The figure shows three views and two pictorial views of one solid part (mm, origin at its lowest corner). Answer the questions. Round coordinates to 2 decimals unless told otherwise and drop trailing zeros. Write each loop counter-clockwise with the first axis right and the second up, starting at its lowest first coordinate (ties: lowest second). Pieces come first, ordered by that corner, then holes. Notation, with made-up numbers: M 74,14 L 98,14 A20 cw 98,33 Z; hole C 73,-10 d11. An arc over 180 degrees is marked long. Answer in a Markdown table with one row per item.
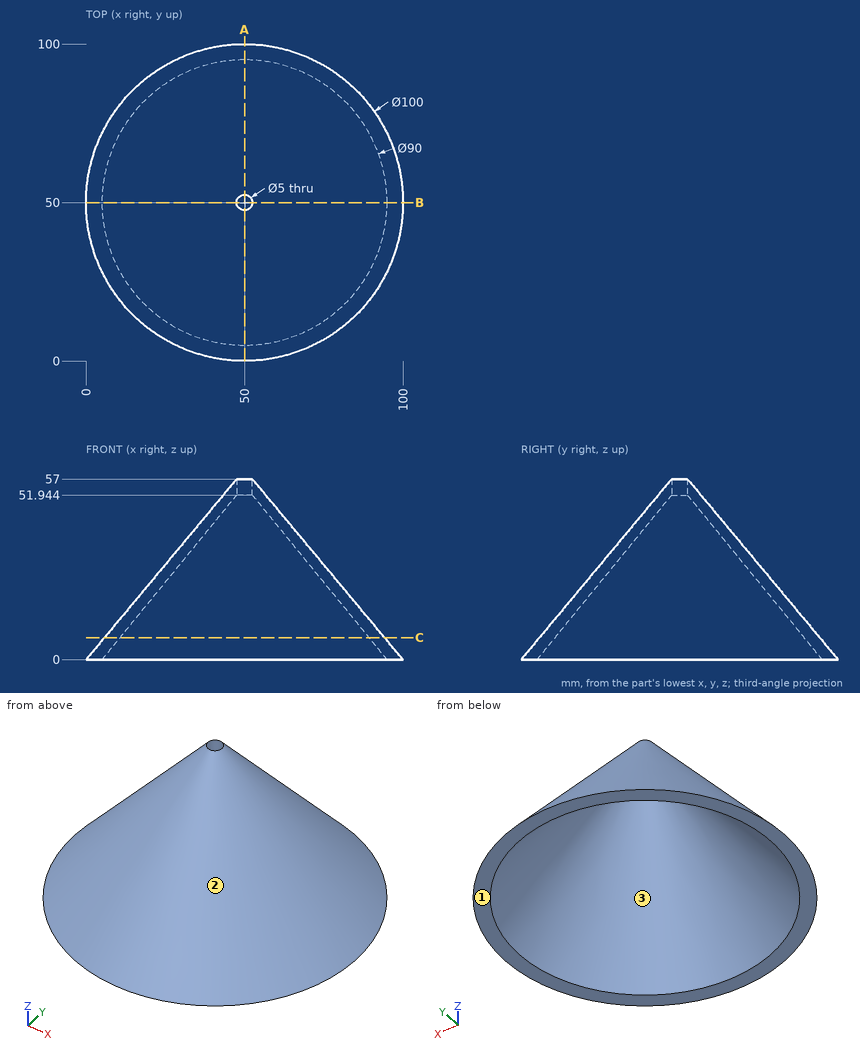
1. Given pin 1 (6 mm diameter, centred on x = 59.5, z = 40, fed in from +Y); pin 2 (3 mm diameter, centred on x = 50, y = 50, fed in from -Z); pin 3 (1 mm diameter, centred on x = 67.5, z = 13, fed in from -Y) (1 decimal); pin 4 (5 mm diameter, centred on x = 63, z = 10.5, fed in from +Y) (1 decimal), each flat-ended and moving along its own axis, determine where each tip first touches the part or whether it passes through.
Calculated:
| item | result |
|---|---|
| pin 1 | stops at y = 67.05 |
| pin 2 | passes through |
| pin 3 | stops at y = 14.4 |
| pin 4 | stops at y = 91.5 |
2. The part is cut by section C-C (z = 7). Determine the outline of the cut face in (x, y) (1 decimal).
Calculated:
| item | result |
|---|---|
| outline | C 50,50 d88.3; hole C 50,50 d78.5 |
3. Determine the mould class of the marked faces 1, 2 and 3 for opening direction Y: released by +Y, released by -Y, zero draft, split by the parting line, or undercut.
Calculated:
| item | result |
|---|---|
| face 1 | zero draft |
| face 2 | split by the parting line |
| face 3 | undercut |
4. The part is cut by section A-A (x = 50). Determine the outline of the cut face in (y, z) (1 decimal), plus the area to 3 significant figures.
Calculated:
| item | result |
|---|---|
| outline | M 0,0 L 5,0 L 47.5,51.9 L 47.5,57 Z; M 52.5,51.9 L 95,0 L 100,0 L 52.5,57 Z |
| area | 500 mm² |
5. Consider line 1 along Y through (x, z) = (50, 53.05); line 2 along X through (y, z) = (50, 53.2) (1 decimal); line 3 along Y through (x, z) = (70, 8) (1 decimal). Determine where each line is inside the solid, lowest interval first. Write a range as from..to.
Calculated:
| item | result |
|---|---|
| line 1 | y = 44.21..47.5, 52.5..55.79 |
| line 2 | x = 44.3..47.5, 52.5..55.7 |
| line 3 | y = 11.6..17.2, 82.8..88.4 |
